```python
from build123d import *

# Parameters (mm, degrees)
F1_DEPTH     = 25.4
F3_DEPTH     = 6.35
F5_DEPTH     = 25.4
F6_W         = 15.08125
F6_H         = 12.7
F7_DEPTH     = 5.3578125
F8_R         = 2.5796875
F9_DEPTH     = 25.4
F12_DEPTH    = 25.4
F13_W        = 19.05
F13_H        = 9.1559581755
F14_DEPTH    = 33.3375
F15_W        = 13.890625
F15_H        = 6.1515625
F16_DEPTH    = 7.9375
F17_W        = 12.7
F17_H        = 1.905
F18_DEPTH    = 6.604
F19_W        = 1.190625
F19_H        = 1.905
F20_DEPTH    = 6.604
F21_W        = 25.003125
F21_H        = 9.921875
F22_DEPTH    = 4.5640625
F24_DEPTH    = 27.94
F25_T1_DEPTH = 59.9739709134
F26_R        = 2.54
F27_R        = 2.54
F28_R        = 5.08


# Not quite as in the source:
# - a fillet or chamfer that OpenCascade refuses, or shapes differently, is made with other operations: its cross-section is extruded or revolved along the edge and cut away or added


with BuildPart() as f1:
    # F0 (on Front) → F1 (new body)
    with BuildSketch(Plane.XZ):
        with BuildLine():
            ThreePointArc((9.525, 43.5474833257), (34.7253859158, 27.9509660298), (44.577, 0))
            ThreePointArc((44.577, 0), (-27.9509660298, -34.7253859158), (-9.525, 43.5474833257))
            Line((-9.525, 43.5474833257), (-9.525, 49.8990418245))
            ThreePointArc((-9.525, 49.8990418245), (-32.3787739113, -39.1440289189), (50.8, 0))
            ThreePointArc((50.8, 0), (39.1440289189, 32.3787739113), (9.525, 49.8990418245))
            Line((9.525, 49.8990418245), (9.525, 43.5474833257))
        make_face()
        with BuildLine():
            ThreePointArc((-9.525, 43.5474833257), (0, 44.577), (9.525, 43.5474833257))
            Line((9.525, 43.5474833257), (9.525, 49.8990418245))
            ThreePointArc((9.525, 49.8990418245), (0, 50.8), (-9.525, 49.8990418245))
            Line((-9.525, 49.8990418245), (-9.525, 43.5474833257))
        make_face()
        with BuildLine():
            ThreePointArc((-9.525, 49.8990418245), (0, 50.8), (9.525, 49.8990418245))
            Line((9.525, 49.8990418245), (9.525, 63.5))
            Line((9.525, 63.5), (-9.525, 63.5))
            Line((-9.525, 63.5), (-9.525, 49.8990418245))
        make_face()
    extrude(amount=F1_DEPTH)

    # F2 (on face) → F3 (cut)
    with BuildSketch(Plane.XZ.offset(25.4)):
        with BuildLine():
            ThreePointArc((0.8929687032, 50.3226047716), (2.6789062266, 50.322604731), (3.571875, 51.8692719891))
            ThreePointArc((3.571875, 51.8692719891), (1.7859375, 53.6552094891), (0, 51.8692719891))
            ThreePointArc((0, 51.8692719891), (0.2392702419, 50.9763032626), (0.8929687032, 50.3226047716))
        make_face()
        with BuildLine():
            ThreePointArc((-0.8929687383, 50.3226047513), (-0.2392702521, 50.976303245), (0, 51.8692719891))
            ThreePointArc((0, 51.8692719891), (-3.3326047479, 52.7622407333), (-0.8929687383, 50.3226047513))
        make_face()
        with BuildLine():
            ThreePointArc((0.8929687032, 50.3226047716), (0.2392702419, 50.9763032626), (0, 51.8692719891))
            ThreePointArc((0, 51.8692719891), (-0.2392702521, 50.976303245), (-0.8929687383, 50.3226047513))
            ThreePointArc((-0.8929687383, 50.3226047513), (-2.03e-08, 50.561875), (0.8929687032, 50.3226047716))
        make_face()
        with BuildLine():
            ThreePointArc((1.7859375, 48.7759375), (1.546667231, 49.6689062734), (0.8929687032, 50.3226047716))
            ThreePointArc((0.8929687032, 50.3226047716), (-2.03e-08, 50.561875), (-0.8929687383, 50.3226047513))
            ThreePointArc((-0.8929687383, 50.3226047513), (-0.8929687558, 47.2292702588), (1.7859375, 48.7759375))
        make_face()
    extrude(amount=-F3_DEPTH, mode=Mode.SUBTRACT)

    # F4 (on Front) → F5 (join)
    with BuildSketch(Plane.XZ):
        with BuildLine():
            Line((-30.48, -65.0875), (30.48, -65.0875))
            Line((30.48, -65.0875), (30.48, -40.64))
            ThreePointArc((30.48, -40.64), (0, -50.8), (-30.48, -40.64))
            Line((-30.48, -40.64), (-30.48, -65.0875))
        make_face()
    extrude(amount=F5_DEPTH)

    # F6 (on face) → F7 (cut)
    with BuildSketch(Plane(origin=(0, 0, -65.0875), x_dir=(1, 0, 0), z_dir=(0, 0, -1))):
        with Locations((20.0421875, 12.7)):
            Rectangle(F6_W, F6_H)
        with Locations((-20.0421875, 12.7)):
            Rectangle(F6_W, F6_H)
    extrude(amount=-F7_DEPTH, mode=Mode.SUBTRACT)

    # F8 (on face) → F9 (cut)
    with BuildSketch(Plane(origin=(0, 0, -59.7296875), x_dir=(1, 0, 0), z_dir=(0, 0, -1))):
        with Locations((21.2328125, 12.7)):
            Circle(F8_R)
        with Locations((-21.2328125, 12.7)):
            Circle(F8_R)
    extrude(amount=-F9_DEPTH, mode=Mode.SUBTRACT)

    # F11 (on offset) → F12 (cut)
    with BuildSketch(Plane.XY.offset(-48.26)):
        Polygon((18.9414536192, -16.66875), (23.5241713808, -16.66875), (25.8155302617, -12.7), (23.5241713808, -8.73125), (18.9414536192, -8.73125), (16.6500947383, -12.7), align=None)
        Polygon((-25.8155302617, -12.7), (-23.5241713808, -16.66875), (-18.9414536192, -16.66875), (-16.6500947383, -12.7), (-18.9414536192, -8.73125), (-23.5241713808, -8.73125), align=None)
    extrude(amount=F12_DEPTH, mode=Mode.SUBTRACT)

    # F13 (on face) → F14 (join)
    with BuildSketch(Plane.XZ.offset(25.4)):
        with Locations((0, 58.9220209122)):
            Rectangle(F13_W, F13_H)
    extrude(amount=F14_DEPTH)

    # F15 (on face) → F16 (cut)
    with BuildSketch(Plane.XZ.offset(58.7375)):
        with Locations((0, 58.6898230745)):
            Rectangle(F15_W, F15_H)
    extrude(amount=-F16_DEPTH, mode=Mode.SUBTRACT)

    # F17 (on face) → F18 (cut)
    with BuildSketch(Plane.XY.offset(63.5)):
        with Locations((0, -49.05375)):
            Rectangle(F17_W, F17_H)
    extrude(amount=-F18_DEPTH, mode=Mode.SUBTRACT)

    # F19 (on face) → F20 (join)
    with BuildSketch(Plane.XY.offset(56.896)):
        with Locations((-2.778125, -49.05375)):
            Rectangle(F19_W, F19_H)
        with Locations((2.778125, -49.05375)):
            Rectangle(F19_W, F19_H)
    extrude(amount=F20_DEPTH)

    # F21 (on face) → F22 (cut)
    with BuildSketch(Plane(origin=(0, 0, -65.0875), x_dir=(1, 0, 0), z_dir=(0, 0, -1))):
        with Locations((0, 12.7)):
            Rectangle(F21_W, F21_H)
    extrude(amount=-F22_DEPTH, mode=Mode.SUBTRACT)

    # F23 (on face) → F24 (cut)
    with BuildSketch(Plane.XZ.offset(25.4)):
        with BuildLine():
            ThreePointArc((44.3832294932, 12.7), (46.1645, 0), (44.3832294932, -12.7))
            Line((44.3832294932, -12.7), (55.8275170624, -12.7))
            Line((55.8275170624, -12.7), (55.8275170624, 12.7))
            Line((55.8275170624, 12.7), (44.3832294932, 12.7))
        make_face()
        with BuildLine():
            Line((-44.3832294932, 12.7), (-55.6385964155, 12.7))
            Line((-55.6385964155, 12.7), (-55.6385964155, -12.7))
            Line((-55.6385964155, -12.7), (-44.3832294932, -12.7))
            ThreePointArc((-44.3832294932, -12.7), (-46.1645, 0), (-44.3832294932, 12.7))
        make_face()
    extrude(amount=-F24_DEPTH, mode=Mode.SUBTRACT)

    # F25: fillet of radius 5.08 on 4 edges, made by hand

    # F25_s2 → F25_t1 (cut)
    with BuildSketch(Plane.XZ.offset(-17.2869854567)):
        with BuildLine():
            ThreePointArc((-44.3832294932, 12.7), (-47.0229133194, 15.4501150062), (-47.0065282778, 19.2620429672))
            Line((-47.0065282778, 19.2620429672), (-47.1005413343, 19.3005670532))
            ThreePointArc((-47.1005413343, 19.3005670532), (-48.3049064769, 16.050199152), (-49.2852622738, 12.7254))
            Line((-49.2852622738, 12.7254), (-49.1868884968, 12.5984))
            ThreePointArc((-49.1868884968, 12.5984), (-46.785058995, 12.5984), (-44.4247765741, 12.6072832266))
            Line((-44.4247765741, 12.6072832266), (-44.3832294932, 12.7))
        make_face()
        with BuildLine():
            ThreePointArc((-47.0065282778, -19.2620429672), (-47.0229133194, -15.4501150062), (-44.3832294932, -12.7))
            Line((-44.3832294932, -12.7), (-44.4247765741, -12.6072832266))
            ThreePointArc((-44.4247765741, -12.6072832266), (-46.785058995, -12.5984), (-49.1868884968, -12.5984))
            Line((-49.1868884968, -12.5984), (-49.2852622738, -12.7254))
            ThreePointArc((-49.2852622738, -12.7254), (-48.3049064769, -16.050199152), (-47.1005413343, -19.3005670532))
            Line((-47.1005413343, -19.3005670532), (-47.0065282778, -19.2620429672))
        make_face()
        with BuildLine():
            ThreePointArc((44.3832294932, -12.7), (47.0229133194, -15.4501150062), (47.0065282778, -19.2620429672))
            Line((47.0065282778, -19.2620429672), (47.1005413343, -19.3005670532))
            ThreePointArc((47.1005413343, -19.3005670532), (48.3049064769, -16.050199152), (49.2852622738, -12.7254))
            Line((49.2852622738, -12.7254), (49.1868884968, -12.5984))
            ThreePointArc((49.1868884968, -12.5984), (46.785058995, -12.5984), (44.4247765741, -12.6072832266))
            Line((44.4247765741, -12.6072832266), (44.3832294932, -12.7))
        make_face()
        with BuildLine():
            ThreePointArc((47.0065282778, 19.2620429672), (47.0229133194, 15.4501150062), (44.3832294932, 12.7))
            Line((44.3832294932, 12.7), (44.4247765741, 12.6072832266))
            ThreePointArc((44.4247765741, 12.6072832266), (46.785058995, 12.5984), (49.1868884968, 12.5984))
            Line((49.1868884968, 12.5984), (49.2852622738, 12.7254))
            ThreePointArc((49.2852622738, 12.7254), (48.3049064769, 16.050199152), (47.1005413343, 19.3005670532))
            Line((47.1005413343, 19.3005670532), (47.0065282778, 19.2620429672))
        make_face()
    extrude(amount=F25_T1_DEPTH, mode=Mode.SUBTRACT)

    # F26
    f26_edges = [f1.edges().sort_by_distance(p)[0] for p in [
        (30.48, -12.7, -65.0875),
        (-30.48, -12.7, -65.0875),
    ]]
    fillet(f26_edges, radius=F26_R)

    # F27
    f27_edges = [f1.edges().sort_by_distance(p)[0] for p in [
        (9.525, -29.36875, 63.5),
        (-9.525, -29.36875, 63.5),
    ]]
    fillet(f27_edges, radius=F27_R)

    # F28
    f28_edges = [f1.edges().sort_by_distance(p)[0] for p in [
        (30.48, -12.7, -40.64),
        (-30.48, -12.7, -40.64),
        (-9.525, -12.7, 49.899042),
        (9.525, -12.7, 49.899042),
    ]]
    fillet(f28_edges, radius=F28_R)


solid = f1.part
```
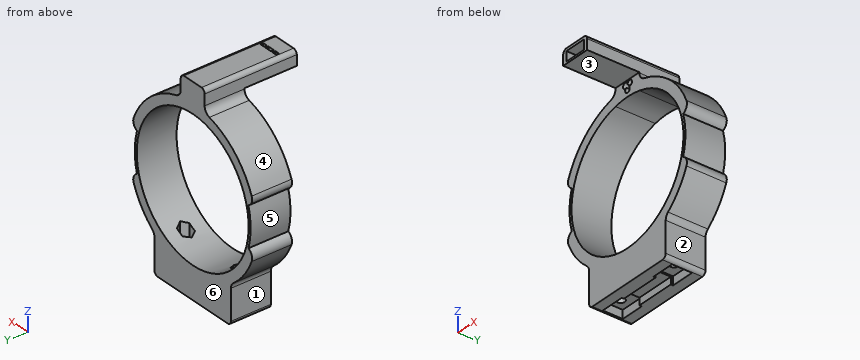
Here's how the part is built. I have some questions about the finished solid (model axes, mm). Face numbers are marked on the shaded views. A direction names the side the tool comes from. Coordinates: 2 decimals unless noted, no trailing zeros. Order: outer loops, then holes, each group sorted by start corner. A loop starts at its lowest first (then second) coordinate and runs counter-clockwise, first axis right, second up. Notation, with made-up numbers: M 14.5,87.5 L 56.5,87.5 A26 ccw 56.5,104.5 Z; hole C 54,83.25 d2. An arc over 180 degrees is marked long. Answer as a JSON object with one key per item and string values. Group by question number.
(1) Suppose I cut it at B-B, the plane y = -54. Please give me the cut outline in (x, z) (3 decimals), then the cut area to 3 significant figures.
(2) I need wall thicknesses on probe 1 along X at (y, z) = (-12.7, -54.5); probe 2 along Z at (x, y) = (0, -8); probe 3 along X at (y, z) = (-4.5, 6.5). Which ranges of each line are inside material? Lowest first, please.
(3) Suppose I cut it at A-A, the plane z = 0. Please give me the cut outline in (x, y).
(4) Suppose I cut it at D-D, the plane y = -22.5. Please give me the cut outline in (x, z) (1 decimal), then the cut area to 3 significant figures.
(5) If we mould it in two halves opening along Z, with no side actions, what happens to the marked faces 4, 5 and 6? For each: released by +Z, released by -Z, zero draft, split by the parting line, or undercut.
(6) For pin 1 (4 mm diameter, centred on y = -25, z = 2.5, fed in from -X); pin 2 (4.5 mm diameter, centred on y = -14, z = -62.5, fed in from +X); pin 3 (2.5 mm diameter, centred on x = 20, z = -63, fed in from -Y), each with a flat end and sliding along its axis, tell me the tip position at first contact or that it passes through.
(7) Suppose I cut it at C-C, the plane z = -53. Please give me the cut outline in (x, y), then the cut area to 3 significant figures.
(8) Which directions (+Z, -Z, +X, -X, +Y, -Y) give clear straight access to the entire face, cutting with the end or side of a thin tool? Please do the marked faces 1, 2 and 3.
Values found:
{
 "1": {"outline": "M -9.525,54.344 L 9.525,54.344 L 9.525,60.96 A2.54 ccw 6.985,63.5 L -6.985,63.5 A2.54 ccw -9.525,60.96 Z; hole M -6.945,55.614 L 6.945,55.614 L 6.945,61.766 L -6.945,61.766 Z", "area": "86.2 mm^2"},
 "2": {"probe 1": "x = -30.48 to -23.81, -18.65 to 18.65, 23.81 to 30.48", "probe 2": "z = -60.52 to -44.58, 44.58 to 63.5", "probe 3": "x = -45.7 to -44.1, 44.1 to 45.7"},
 "3": {"outline": "M -46.16,-25.4 L -44.58,-25.4 L -44.58,0 L -46.16,0 Z; M 44.58,-25.4 L 46.16,-25.4 L 46.16,0 L 44.58,0 Z"},
 "4": {"outline": "M -47,-19.3 A50.8 ccw -32.3,-39.2 A5.1 cw -30.5,-43.1 L -30.5,-62.5 A2.5 ccw -27.9,-65.1 L 27.9,-65.1 A2.5 ccw 30.5,-62.5 L 30.5,-43.1 A5.1 cw 32.3,-39.2 A50.8 ccw 47,-19.3 A5.1 ccw 44.4,-12.7 A46.2 ccw 44.4,12.7 A5.1 ccw 47,19.3 A50.8 ccw 13.3,49 A5.1 cw 9.5,53.9 L 9.5,61 A2.5 ccw 7,63.5 L -7,63.5 A2.5 ccw -9.5,61 L -9.5,53.9 A5.1 cw -13.3,49 A50.8 ccw -47,19.3 A5.1 ccw -44.4,12.7 A46.2 ccw -44.4,-12.7 A5.1 ccw Z; hole C 0,0 d89.2; hole M -0.9,50.3 A1.8 ccw long 0.9,50.3 A1.8 ccw long 0,51.9 A1.8 ccw long Z", "area": "2,880 mm^2"},
 "5": {"face 4": "released by +Z", "face 5": "undercut", "face 6": "zero draft"},
 "6": {"pin 1": "stops at x = -46.16", "pin 2": "stops at x = 30.48", "pin 3": "stops at y = -25.4"},
 "7": {"outline": "M -30.48,-25.4 L 30.48,-25.4 L 30.48,0 L -30.48,0 Z; hole C -21.23,-12.7 d5.16; hole C 21.23,-12.7 d5.16", "area": "1,510 mm^2"},
 "8": {"face 1": "-Z, -X, +Y, -Y", "face 2": "-Z, +X, +Y, -Y", "face 3": "-Z, +X, -X, -Y"}
}
